Part model, mm, in its own coordinate system. A direction names the side the tool comes from. Coordinates: 2 decimals unless noted, no trailing zeros. Order: outer loops, then holes, each group sorted by start corner. A loop starts at its lowest first (then second) coordinate and runs counter-clockwise, first axis right, second up.
from build123d import *

# Parameters (mm, degrees)
SKETCH2_W           = 70.6
SKETCH2_H           = 55.3
BOSS_EXTRUDE1_DEPTH = 11
SHELL1_T            = 1.6
FILLET1_R           = 2.5
SKETCH2_4_R         = 2.6
SKETCH2_4_R_2       = 1.6
BOSS_EXTRUDE2_DEPTH = 10
CUT_EXTRUDE1_DEPTH  = 3
CUT_EXTRUDE2_DEPTH  = 3
SKETCH8_W           = 48.24
SKETCH8_H           = 3.41
SKETCH8_W_2         = 39.1
CUT_EXTRUDE3_DEPTH  = 1.8
CUT_EXTRUDE4_DEPTH  = 3.5
CHAMFER1_SIZE       = 0.45


with BuildPart() as part:
    # Sketch2 → Boss-Extrude1 (new body)
    with BuildSketch(Plane(origin=(0, 0, 0), x_dir=(1, 0, 0), z_dir=(0, 1, 0))):
        with Locations((34.3, 26.65)):
            Rectangle(SKETCH2_W, SKETCH2_H)
    extrude(amount=BOSS_EXTRUDE1_DEPTH)

    # Shell1
    shell1_openings = [part.faces().sort_by_distance(p)[0] for p in [
        (34.3, 11, -26.65),
    ]]
    offset(amount=SHELL1_T, openings=shell1_openings, kind=Kind.INTERSECTION)

    # Fillet1
    # the kernel refuses this fillet: 2.5 mm, written as the material it takes off along each edge
    with BuildSketch(Plane(origin=(-2.6, 17.25, 2.6), x_dir=(1, 0, 0), z_dir=(0, -1, 0)), Plane(origin=(71.2, 17.25, 2.6), x_dir=(0, 0, -1), z_dir=(0, -1, 0)), Plane(origin=(71.2, 17.25, -55.9), x_dir=(-1, 0, 0), z_dir=(0, -1, 0)), Plane(origin=(-2.6, -7.85, -55.9), x_dir=(1, 0, 0), z_dir=(0, 1, 0))) as fillet1_piece_1:
        with BuildLine():
            CenterArc((FILLET1_R, -FILLET1_R), FILLET1_R, 90, 90)
            Line((0, -FILLET1_R), (0, 0))
            Line((0, 0), (FILLET1_R, 0))
        make_face()
    extrude(amount=25.1, mode=Mode.SUBTRACT)

    # Sketch2<4> → Boss-Extrude2 (add)
    # profile 1 of 3: a face of its own
    with BuildSketch(Plane(origin=(0, 0, 0), x_dir=(1, 0, 0), z_dir=(0, 1, 0))):
        with Locations(Location((66.1, 17.8, 0), (0, 0, 90))):
            Circle(SKETCH2_4_R)
        with Locations(Location((66.1, 17.8, 0), (0, 0, 270))):
            Circle(SKETCH2_4_R_2, mode=Mode.SUBTRACT)
    # profile 2 of 3: a face of its own
    with BuildSketch(Plane(origin=(0, 0, 0), x_dir=(1, 0, 0), z_dir=(0, 1, 0))):
        with Locations(Location((14, 50.8, 0), (0, 0, 90))):
            Circle(SKETCH2_4_R)
        with Locations(Location((14, 50.8, 0), (0, 0, 270))):
            Circle(SKETCH2_4_R_2, mode=Mode.SUBTRACT)
    # profile 3 of 3: a face of its own
    with BuildSketch(Plane(origin=(0, 0, 0), x_dir=(1, 0, 0), z_dir=(0, 1, 0))):
        with Locations(Location((66.1, 45.7, 0), (0, 0, 90))):
            Circle(SKETCH2_4_R)
        with Locations(Location((66.1, 45.7, 0), (0, 0, 270))):
            Circle(SKETCH2_4_R_2, mode=Mode.SUBTRACT)
    extrude(amount=BOSS_EXTRUDE2_DEPTH)

    # Sketch4 → Cut-Extrude1 (cut)
    with BuildSketch(Plane.ZY.offset(2.6)):
        with BuildLine():
            Line((-21.810563814, 11), (-21.810563814, 5.78))
            ThreePointArc((-21.810563814, 5.78), (-21.530873699, 5.10266948), (-20.854775908, 4.820012494))
            Line((-20.854775908, 4.820012494), (-9.735787906, 4.820012494))
            ThreePointArc((-9.735787906, 4.820012494), (-9.058457386, 5.101442143), (-8.78, 5.78))
            Line((-8.78, 5.78), (-8.78, 11))
            Line((-8.78, 11), (-21.810563814, 11))
        make_face()
    extrude(amount=-CUT_EXTRUDE1_DEPTH, mode=Mode.SUBTRACT)

    # Sketch6 → Cut-Extrude2 (cut)
    with BuildSketch(Plane.ZY.offset(2.6)):
        with BuildLine():
            Line((-50.64, 11), (-50.64, 5.846332149))
            ThreePointArc((-50.64, 5.846332149), (-50.33827519, 5.142948487), (-49.627556174, 4.858932788))
            Line((-49.627556174, 4.858932788), (-41.634891875, 4.858932788))
            ThreePointArc((-41.634891875, 4.858932788), (-40.924172858, 5.142948487), (-40.622448048, 5.846332149))
            Line((-40.622448048, 5.846332149), (-40.622448048, 11))
            Line((-40.622448048, 11), (-50.64, 11))
        make_face()
    extrude(amount=-CUT_EXTRUDE2_DEPTH, mode=Mode.SUBTRACT)

    # Sketch8 → Cut-Extrude3 (cut)
    with BuildSketch(Plane.XZ.offset(1.6)):
        with Locations((41.21, -2.525)):
            Rectangle(SKETCH8_W, SKETCH8_H)
        with Locations((45.78, -50.785)):
            Rectangle(SKETCH8_W_2, SKETCH8_H)
    extrude(amount=-CUT_EXTRUDE3_DEPTH, mode=Mode.SUBTRACT)

    # Sketch10 → Cut-Extrude4 (cut)
    with BuildSketch(Plane(origin=(0, -1.6, 0), x_dir=(-1, 0, 0), z_dir=(0, -1, 0))):
        Polygon((-2.5, 26.65), (0, 26.65), (-5.685748819, 11.028533507), (-8.185748819, 11.028533507), align=None)
        with BuildLine():
            Line((-2.5, 26.65), (0, 26.65))
            ThreePointArc((0, 26.65), (-1.25, 27.9), (-2.5, 26.65))
        make_face()
        with BuildLine():
            Line((-2.5, 41.272108294), (-2.5, 34.309766621))
            ThreePointArc((-2.5, 34.309766621), (-1.25, 33.059766621), (0, 34.309766621))
            Line((0, 34.309766621), (0, 41.272108294))
            ThreePointArc((0, 41.272108294), (-1.25, 42.522108294), (-2.5, 41.272108294))
        make_face()
        Polygon((-15.685748819, 11.028533507), (-10, 26.65), (-12.5, 26.65), (-18.185748819, 11.028533507), align=None)
        Polygon((-12.5, 26.65), (-10, 26.65), (-15.685748819, 42.271466493), (-18.185748819, 42.271466493), align=None)
        Polygon((-25.685748819, 11.028533507), (-20, 26.65), (-22.5, 26.65), (-28.185748819, 11.028533507), align=None)
        Polygon((-22.5, 26.65), (-20, 26.65), (-25.685748819, 42.271466493), (-28.185748819, 42.271466493), align=None)
        Polygon((-35.685748819, 11.028533507), (-30, 26.65), (-32.5, 26.65), (-38.185748819, 11.028533507), align=None)
        Polygon((-32.5, 26.65), (-30, 26.65), (-35.685748819, 42.271466493), (-38.185748819, 42.271466493), align=None)
        Polygon((-45.685748819, 11.028533507), (-40, 26.65), (-42.5, 26.65), (-48.185748819, 11.028533507), align=None)
        Polygon((-42.5, 26.65), (-40, 26.65), (-45.685748819, 42.271466493), (-48.185748819, 42.271466493), align=None)
        Polygon((-55.685748819, 11.028533507), (-50, 26.65), (-52.5, 26.65), (-58.185748819, 11.028533507), align=None)
        Polygon((-52.5, 26.65), (-50, 26.65), (-55.685748819, 42.271466493), (-58.185748819, 42.271466493), align=None)
    extrude(amount=-CUT_EXTRUDE4_DEPTH, mode=Mode.SUBTRACT)

    # Chamfer1
    chamfer1_edges = [part.edges().sort_by_distance(p)[0] for p in [
        (-2.6, -1.6, -26.65),
        (34.3, -1.6, -55.9),
        (71.2, -1.6, -26.65),
        (34.3, -1.6, 2.6),
        (70.467766953, -1.6, 1.867766953),
        (70.467766953, -1.6, -55.167766953),
        (-1.867766953, -1.6, 1.867766953),
        (-1.867766953, -1.6, -55.167766953),
    ]]
    chamfer(chamfer1_edges, length=CHAMFER1_SIZE)


solid = part.part
Q1. Which spindle directions (+Z, -Z, +X, -X, +Y, -Y) get a long thin tool onto all of the face, cutting with end or side? Do faces 1 (the face through (52.803, -0.811, -34.351)), 2 (the face through (-1.65, -1.48, -54.92)), 3 (the face through (14.07, 4.93, -52.4)). Say none if no direction does.
Results list:
face 1: +Y, -Y
face 2: -Z, -X, -Y
face 3: +Y
Q2. Cut at A-A on y = 3.5. Write the cut outline in (x, z).
Results list:
outline: (-2.6, -53.4) arc R2.5 ccw to (-0.1, -55.9) - (68.7, -55.9) arc R2.5 ccw to (71.2, -53.4) - (71.2, 0.1) arc R2.5 ccw to (68.7, 2.6) - (-0.1, 2.6) arc R2.5 ccw to (-2.6, 0.1) - close; circle Ø5.2 at (14, -50.8); circle Ø5.2 at (66.1, -45.7); circle Ø5.2 at (66.1, -17.8); hole (-1, -54.3) - (69.6, -54.3) - (69.6, 1) - (-1, 1) - close; hole circle Ø3.2 at (14, -50.8); hole circle Ø3.2 at (66.1, -45.7); hole circle Ø3.2 at (66.1, -17.8)
Q3. Mould opens along X. For faces 4 (the face through (70.448, 5.01, -55.187)), 5 (the face through (1.28, -0.81, -33.06)), 6 (the face through (34, 5, -55.9)) say: pulls with the +X half, pulls with the -X half, needs draft (parallel to the pull), parting line crosses it, or undercut.
Results list:
face 4: pulls with the +X half
face 5: undercut
face 6: needs draft
Q4. Cut at B-B on x = 60.5. Write the cut outline in (y, z).
Results list:
outline: (-1.6, -55.45) - (-1.15, -55.9) - (11, -55.9) - (11, -54.3) - (0, -54.3) - (0, -52.49) - (-1.6, -52.49) - close; (-1.6, -49.08) - (0, -49.08) - (0, -4.23) - (-1.6, -4.23) - close; (-1.6, -0.82) - (0, -0.82) - (0, 1) - (11, 1) - (11, 2.6) - (-1.15, 2.6) - (-1.6, 2.15) - close
Q5. Cut at D-D on z = -25.5. Count the separate pieces of the cut face and the enclosed holes in it, and give its area (3 significant figures).
Results list:
separate pieces: 7
enclosed holes: 0
area: 129 mm2
Q6. Pin check, flat tips, straight feed: pin 1 Ø1.5 at (x, z) = (8, -21) entering from +Y; pin 2 Ø1.3 at (x, y) = (-1.5, 8) entering from -Z; pin 3 Ø5.5 at (x, z) = (14, -51) entering from +Y. Stop position of each tip, or through.
Results list:
pin 1: stops at y = 0
pin 2: stops at z = -55.78
pin 3: stops at y = 10
Q7. Cut at C-C on z = -45.7. Write the cut outline in (x, y).
Results list:
outline: (-2.6, -1.15) - (-2.15, -1.6) - (70.75, -1.6) - (71.2, -1.15) - (71.2, 11) - (69.6, 11) - (69.6, 0) - (68.7, 0) - (68.7, 10) - (67.7, 10) - (67.7, 0) - (64.5, 0) - (64.5, 10) - (63.5, 10) - (63.5, 0) - (-1, 0) - (-1, 4.86) - (-2.6, 4.86) - close
Q8. Wall check: line 1 along Z through (x, y) = (66.1, 7.5); line 2 along Z through (x, y) = (59, 6.25); line 3 along X through (y, z) = (8, -17.8). Give the ranges that are in metal, low to high.
Results list:
line 1: z = -55.9 to -54.3, -48.3 to -47.3, -44.1 to -43.1, -20.4 to -19.4, -16.2 to -15.2, 1 to 2.6
line 2: z = -55.9 to -54.3, 1 to 2.6
line 3: x = 63.5 to 64.5, 67.7 to 68.7, 69.6 to 71.2
